Design review of the part built by this model. Coordinates are the model's own, in mm. Face numbers are marked on the shaded views. A direction names the side the tool comes from. Round coordinates to 2 decimals unless told otherwise and drop trailing zeros. Write each loop counter-clockwise with the first axis right and the second up, starting at its lowest first coordinate (ties: lowest second). Pieces come first, ordered by that corner, then holes. Notation, with made-up numbers: M -4.75,0.25 L 38.25,0.25 A15 cw 38.25,23.25 Z; hole C -1,80 d3. An arc over 180 degrees is marked long. Use CSV: the item, a comma, the result in double quotes.
from build123d import *

# Parameters (mm, degrees)
F1_DEPTH = 4
F2_DEPTH = 2


# Not quite as in the source:
# - a feature names something its author has since deleted; it is built from what else it names


with BuildPart() as f1:
    # F0 (on Front) → F1 (new body)
    with BuildSketch(Plane.XZ):
        with BuildLine():
            ThreePointArc((-69.017292897, 29.3982457694), (-68.3268421331, 27.2084157133), (-66.290176034, 26.1481944472))
            Line((-66.290176034, 26.1481944472), (-65.4847666663, 26.0777302572))
            ThreePointArc((-65.4847666663, 26.0777302572), (-63.2535898646, 26.8035186892), (-62.2272009721, 28.913363378))
            Line((-62.2272009721, 28.913363378), (-61.5372568785, 35.1033145465))
            Line((-61.5372568785, 35.1033145465), (-53.1481667688, 34.3565562926))
            Line((-53.1481667688, 34.3565562926), (-54.3320948451, 17.7259296179))
            Line((-54.3320948451, 17.7259296179), (-43.1615771204, 6.577645293))
            ThreePointArc((-43.1615771204, 6.577645293), (-35.1559477392, 3.3688057895), (-27.2990026255, 6.9262158348))
            Line((-27.2990026255, 6.9262158348), (-3.5743886341, 49.0892314075))
            ThreePointArc((-3.5743886341, 49.0892314075), (-6.738115065, 55.6702900526), (-13.9632260986, 54.6132808892))
            Line((-13.9632260986, 54.6132808892), (-36.8751008064, 13.8946529478))
            Line((-36.8751008064, 13.8946529478), (-46.112828888, 19.5994470268))
            Line((-46.112828888, 19.5994470268), (-45.1602484403, 32.9947581421))
            ThreePointArc((-45.1602484403, 32.9947581421), (-46.4251891271, 36.9862585641), (-50.0833280385, 39.0234552324))
            Line((-50.0833280385, 39.0234552324), (-64.8513762012, 40.3222609912))
            ThreePointArc((-64.8513762012, 40.3222609912), (-67.0146267862, 39.6550864105), (-68.0957389782, 37.666124007))
            Line((-68.0957389782, 37.666124007), (-69.017292897, 29.3982457694))
        make_face()
        Polygon((-9.9778777986, 47.8288231225), (-31.1708185564, 10.1650579072), (-34.5696903843, 12.0775615796), (-13.3767496278, 49.7413267956), align=None, mode=Mode.SUBTRACT)
    extrude(amount=F1_DEPTH)

    # F0 (on Front) → F2 (join)
    with BuildSketch(Plane.XZ):
        Polygon((-34.5696903843, 12.0775615796), (-31.1708185564, 10.1650579072), (-9.9778777986, 47.8288231225), (-13.3767496278, 49.7413267956), align=None)
    extrude(amount=F2_DEPTH)


solid = f1.part
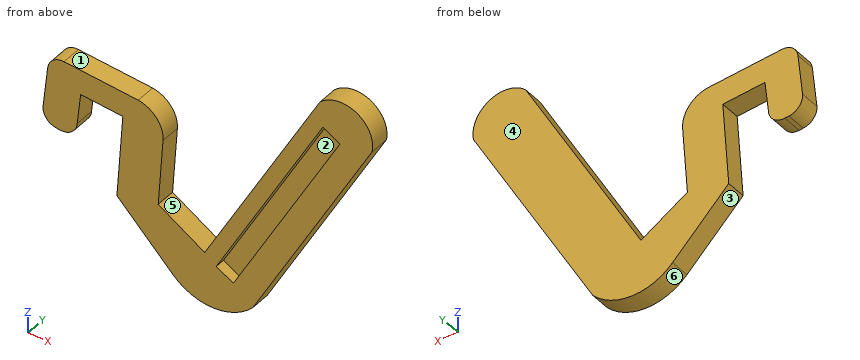
1) Machinability: for the marked faces 1, 2 and 3, which of the approach directions +Z, -Z, +X, -X, +Y, -Y give a long, thin tool a straight path to every point of the face, cutting with its end or side? Answer none if there is none.
Answers:
face 1,"+Z, +Y, -Y"
face 2,"-Y"
face 3,"-Z, -X, +Y, -Y"
2) Add section B-B on z = 25. Write out the cut boundary in (x, y), then the cut area to 3 significant figures.
Answers:
outline,"M -53.81,-4 L -45.73,-4 L -45.73,0 L -53.81,0 Z; M -30.63,-4 L -27.3,-4 L -27.3,-2 L -22.82,-2 L -22.82,-4 L -17.13,-4 L -17.13,0 L -30.63,0 Z"
area,"77.4 mm²"
3) Wall thickness on line 1 along X through (y, z) = (-2.3, 26); line 2 along Y through (x, z) = (-15, 44); line 3 along X through (y, z) = (-3.1, 41.5): over which ranges is each line inside the solid? List them lowest first. Write a range as [from, to].
Answers:
line 1,"[-53.74, -45.66], [-30.06, -26.74], [-22.26, -16.57]"
line 2,"[-2, 0]"
line 3,"[-21.34, -18.01], [-13.54, -7.84]"
4) For pin 1 Ø1 at (x, y) = (-50.5, -2.5) entering from -Z; pin 2 Ø2 at (x, z) = (-14, 46) entering from -Y; pin 3 Ø1 at (y, z) = (-2, 49) entering from +X, all flat-tipped, find the tip position at first contact; note any pin that passes through.
Answers:
pin 1,"z = 13.4"
pin 2,"y = -2"
pin 3,"x = -3.51"
5) The part is to be moulded in two halves that separate along X. For the marked faces 4, 5 and 6, say which applies: released by +X, released by -X, zero draft, split by the parting line, or undercut.
Answers:
face 4,"zero draft"
face 5,"undercut"
face 6,"split by the parting line"
6) Add section A-A on y = -3.25. Write out the cut boundary in (x, z).
Answers:
outline,"M -69.02,29.4 A3 ccw -66.29,26.15 L -65.48,26.08 A3 ccw -62.23,28.91 L -61.54,35.1 L -53.15,34.36 L -54.33,17.73 L -43.16,6.58 A10.99 ccw -27.3,6.93 L -3.57,49.09 A6.16 ccw -13.96,54.61 L -36.88,13.89 L -46.11,19.6 L -45.16,32.99 A5.67 ccw -50.08,39.02 L -64.85,40.32 A3 ccw -68.1,37.67 Z; hole M -34.57,12.08 L -31.17,10.17 L -9.98,47.83 L -13.38,49.74 Z"
7) Add section D-D on z = 44. Write out the cut boundary in (x, y).
Answers:
outline,"M -19.94,-4 L -16.61,-4 L -16.61,-2 L -12.13,-2 L -12.13,-4 L -6.44,-4 L -6.44,0 L -19.94,0 Z"
8) Add section C-C on x = -48.5. Write out the cut boundary in (y, z).
Answers:
outline,"M -4,11.91 L 0,11.91 L 0,38.58 L -4,38.58 Z"
